Work out the finished part from the listing and answer in its coordinate system (mm). Face numbers are marked on the shaded views. Round coordinates to 2 decimals unless told otherwise and drop trailing zeros. Loops run counter-clockwise (first coordinate to the right, second up) from the corner with the lowest first, then second, coordinate; pieces in that order, holes last. Notation, with made-up numbers: M -16,25 L 37,25 A20 cw 37,30 Z; hole C -32,0.25 d1. An arc over 180 degrees is marked long. One line per item, written item: value.
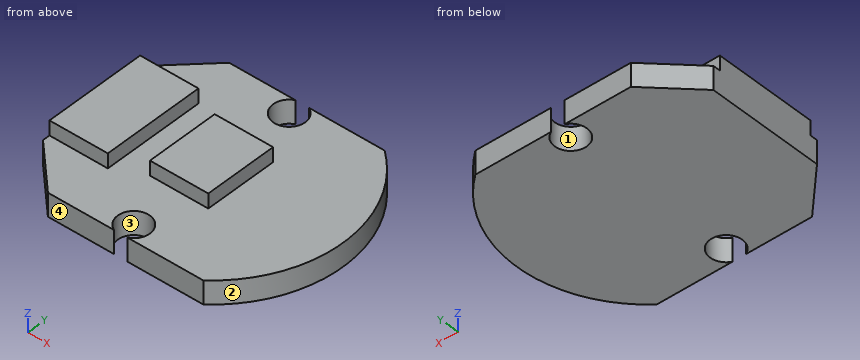
```python
from build123d import *

# Parameters (mm, degrees)
SALIENTE_EXTRUIR1_DEPTH = 1.6
CROQUIS2_R              = 1.1
CORTAR_EXTRUIR2_DEPTH   = 12.513470372
CROQUIS3_W              = 4
CROQUIS3_H              = 5
CROQUIS3_H_2            = 7
SALIENTE_EXTRUIR2_DEPTH = 1


with BuildPart() as part:
    # Croquis1 → Saliente-Extruir1 (new body)
    with BuildSketch(Plane.XY):
        with BuildLine():
            Line((5.656854249, 7), (-5, 7))
            Line((-5, 7), (-8, 4))
            Line((-8, 4), (-8, -4))
            Line((-8, -4), (-5, -7))
            Line((-5, -7), (5.656854249, -7))
            ThreePointArc((5.656854249, -7), (9, 0), (5.656854249, 7))
        make_face()
    extrude(amount=SALIENTE_EXTRUIR1_DEPTH)

    # Croquis2 → Cortar-Extruir2 (cut, through all)
    with BuildSketch(Plane.XY.offset(1.6)):
        with Locations((0, 6)):
            Circle(CROQUIS2_R)
        with Locations((0, -6)):
            Circle(CROQUIS2_R)
    extrude(amount=-CORTAR_EXTRUIR2_DEPTH, mode=Mode.SUBTRACT)

    # Croquis3 → Saliente-Extruir2 (add)
    with BuildSketch(Plane.XY.offset(1.6)):
        Rectangle(CROQUIS3_W, CROQUIS3_H)
        with Locations((-6, 0)):
            Rectangle(CROQUIS3_W, CROQUIS3_H_2)
    extrude(amount=SALIENTE_EXTRUIR2_DEPTH)


solid = part.part
```
1) Find section B-B (y = 0). Give the vertices of the cut face in (x, z), then the cut area to 3 significant figures.
Check values:
outline: M -8,0 L 9,0 L 9,1.6 L 2,1.6 L 2,2.6 L -2,2.6 L -2,1.6 L -4,1.6 L -4,2.6 L -8,2.6 Z
area: 35.2 mm2
2) Find the intervals of material crossed by probe 1 along X at (y, z) = (1.5, 1.8); probe 2 along Z at (x, y) = (4.5, -1.5); probe 3 along Y at (x, z) = (0, 0.8), in increasing order. Write a range as from..to.
Check values:
probe 1: -8..-4, -2..2
probe 2: 0..1.6
probe 3: -4.9..4.9
3) Find section A-A (z = 2). Give the vertices of the cut face in (x, y).
Check values:
outline: M -8,-3.5 L -4,-3.5 L -4,3.5 L -8,3.5 Z; M -2,-2.5 L 2,-2.5 L 2,2.5 L -2,2.5 Z
4) Each of these flat-tipped pins is pushed along its axis until it touches: pin 1 (1 mm diameter, centred on y = -5.5, z = 1.5, fed in from -X); pin 2 (0.5 mm diameter, centred on y = -0.5, z = 2, fed in from +X); pin 3 (1.3 mm diameter, centred on x = 0, y = 6, fed in from -Z); pin 4 (0.5 mm diameter, centred on x = -1, z = 2, fed in from +Y). Where does it stop, or does it pass through?
Check values:
pin 1: x = -7
pin 2: x = 2
pin 3: through
pin 4: y = 2.5
5) Find section D-D (x = 0). Give the vertices of the cut face in (y, z), then the cut area to 3 significant figures.
Check values:
outline: M -4.9,0 L 4.9,0 L 4.9,1.6 L 2.5,1.6 L 2.5,2.6 L -2.5,2.6 L -2.5,1.6 L -4.9,1.6 Z
area: 20.7 mm2
6) Find section C-C (y = 6). Give the vertices of the cut face in (x, z), then the cut area to 3 significant figures.
Check values:
outline: M -6,0 L -1.1,0 L -1.1,1.6 L -6,1.6 Z; M 1.1,0 L 6.71,0 L 6.71,1.6 L 1.1,1.6 Z
area: 16.8 mm2
7) The mould has two halves that part along Y. Classify the marked faces 1, 2, 3 and 4: +Y half, -Y half, draft (parallel to the pull), parting line (faces both ways), or undercut.
Check values:
face 1: undercut
face 2: parting line
face 3: undercut
face 4: -Y half
